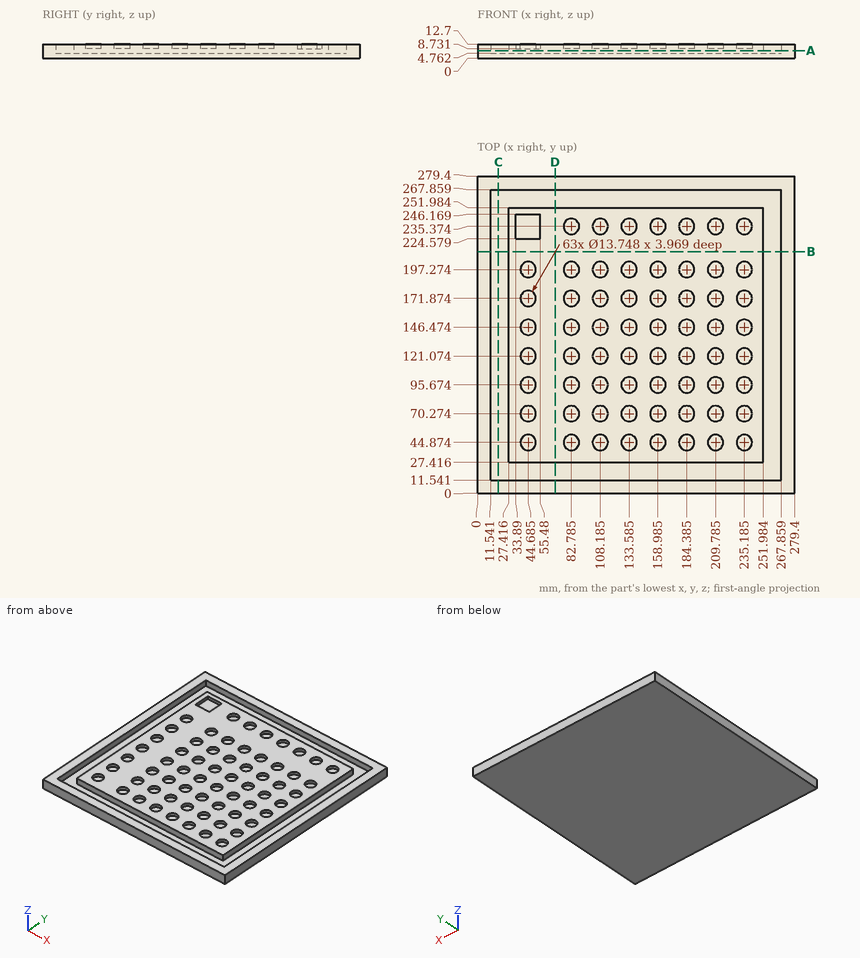
Here's the drawing with two shaded views (mm, measured from the low corner). I have some questions. Coordinates: 2 decimals unless noted, no trailing zeros. Write each loop counter-clockwise with the first axis right and the second up, starting at its lowest first coordinate (ties: lowest second). Pieces come first, ordered by that corner, then holes.
Item 1: I want a section at A-A on z = 6.75. Write out the boundary of the cut face in (x, y).
Item 2: I want a section at C-C on x = 18.5. Write out the boundary of the cut face in (y, z), and give its area (3 significant figures).
Item 3: I want a section at B-B on y = 213. Write out the boundary of the cut face in (x, z), and give its area (3 significant figures).
Item 4: Will this pin go through, and if not, where does the flat tip stop? pin 1 (7 mm diameter, centred on x = 105.5, y = 198, fed in from +Z).
Item 5: If I drill on line 1 (X direction, y = 67, z = 8.25); line 2 (X direction, y = 260, z = 7.5), over which ranges is the centre line in solid material (lowest first)?
Findings below:
1. outline: (0, 0) - (279.4, 0) - (279.4, 279.4) - (0, 279.4) - close; (27.42, 27.42) - (251.98, 27.42) - (251.98, 251.98) - (27.42, 251.98) - close; hole (11.54, 11.54) - (267.86, 11.54) - (267.86, 267.86) - (11.54, 267.86) - close
2. outline: (0, 0) - (279.4, 0) - (279.4, 12.7) - (267.86, 12.7) - (267.86, 4.76) - (11.54, 4.76) - (11.54, 12.7) - (0, 12.7) - close
2. area: 1,510 mm2
3. outline: (0, 0) - (279.4, 0) - (279.4, 12.7) - (267.86, 12.7) - (267.86, 4.76) - (251.98, 4.76) - (251.98, 12.7) - (27.42, 12.7) - (27.42, 4.76) - (11.54, 4.76) - (11.54, 12.7) - (0, 12.7) - close
3. area: 3,300 mm2
4. pin 1: stops at z = 8.73
5. line 1: x = 0 to 11.54, 27.42 to 251.98, 267.86 to 279.4
5. line 2: x = 0 to 11.54, 267.86 to 279.4
